For this review, take the finished solid that the model builds, in its own axes (mm). Face numbers are marked on the shaded views. A direction names the side the tool comes from. Round coordinates to 2 decimals unless told otherwise and drop trailing zeros. Loops run counter-clockwise (first coordinate to the right, second up) from the corner with the lowest first, then second, coordinate; pieces in that order, holes last.
1) Insertion check: pin 1 (18 mm diameter, centred on x = 24, z = -19, fed in from -Y). The pin has a flat end and moves straight along its axis. Give the tip position at first contact, or say it passes through.
2) Take a section at A-A (x = 32). State the section outline as (y, z) points.
3) Wall thickness on L1, parallel to Z at x = 24, y = 8; L2, parallel to X at y = 12, z = -17.5; L3, parallel to X at y = 9.25, z = -11: over which ranges is each line inside the solid? List them lowest first.
4) Take a section at B-B (z = -11). State the section outline as (x, y) points, then the cut area to 3 significant figures.
5) Tool access review of the marked faces 1 and 2: name each direction out of +Z, -Z, +X, -X, +Y, -Y from which nothing blocks a thin tool from reaching the whole face with its end or side.
6) Mouldability with a two-part tool opening along X and no side actions: class the marked faces 3, 4 and 5 as pulls with the +X half, pulls with the -X half, needs draft (parallel to the pull), parting line crosses it, or undercut.
7) Take a section at D-D (z = -21). State the section outline as (x, y) points, then the cut area to 3 significant figures.
8) Take a section at C-C (y = 4.75). State the section outline as (x, z) points.
Autodesk Inventor part; units mm, degrees
ref_plane "YZ Plane" through (0, 0, 0) normal (1, 0, 0) x (0, 1, 0)
ref_plane "XZ Plane" through (0, 0, 0) normal (0, 1, 0) x (-1, 0, 0)
ref_plane "XY Plane" through (0, 0, 0) normal (0, 0, 1) x (1, 0, 0)
sketch "Sketch1" plane through (0, 0, 0) normal (0, 1, 0) x (-1, 0, 0)
  line L0 (-84, -3) -> (-84, -35)
  line L1 (-80, -39) -> (-24, -39)
  line L2 (-52, -9) -> (-52, -23)
  line L3 (-56, -27) -> (-68, -27)
  line L4 (-72, -23) -> (-72, -3)
  line L5 (-24, 1) -> (-42, 1)
  line L6 (-76, 1) -> (-80, 1)
  arc A0 (-80, 1) -> (-84, -3) centre (-80, -3) ccw
  arc A1 (-72, -3) -> (-76, 1) centre (-76, -3) ccw
  arc A2 (-84, -35) -> (-80, -39) centre (-80, -35) ccw
  arc A3 (-72, -23) -> (-68, -27) centre (-68, -23) ccw
  arc A4 (-56, -27) -> (-52, -23) centre (-56, -23) ccw
  arc A5 (-24, -39) -> (-24, 1) centre (-24, -19) ccw
  arc A6 (-42, 1) -> (-52, -9) centre (-42, -9) ccw
  line L7 (-4, -19) -> (-4, -49)
  line L8 (-4, -49) -> (-84, -49)
  line L9 (-84, -49) -> (-84, -35)
  point P0 (-84, -39)
  point P1 (-52, -27)
  point P2 (-52, 1)
  point P3 (-72, -27)
  dimension "d2" = 20
  dimension "d4" = 12
  dimension "d6" = 40
  dimension "d9" = 40
  dimension "d24" = 4
  dimension "d25" = 10
  dimension "d26" = 28
  dimension "d27" = 12
  dimension "d32" = 30
extrude "Extrusion1" add sketch "Sketch1" along normal blind 12.7
sketch "Sketch2" plane through (0, 12.7, 0) normal (0, 1, 0) x (1, 0, 0)
  circle A0 centre (24, 19) radius 7
  arc A1 (4, 19) -> (24, -1) centre (24, 19) ccw
  circle A2 centre (32, 27) radius 2.05
  circle A3 centre (16, 27) radius 2.05
  circle A4 centre (16, 11) radius 2.05
  circle A5 centre (32, 11) radius 2.05
  point P0 (0, 0)
  point P1 (24, 39)
  dimension "d13" = 14
  dimension "d14" = 4.1
  dimension "d15" = 4.1
  dimension "d16" = 4.1
  dimension "d17" = 4.1
  dimension "d18" = 16
  dimension "d19" = 16
  dimension "d20" = 8
  dimension "d21" = 8
extrude "Extrusion2" cut sketch "Sketch2" against normal through all
fillet "Fillet1" radius 5 2 edges at (84, 6.35, -49) (4, 6.35, -49)
properties part number "platform hook"
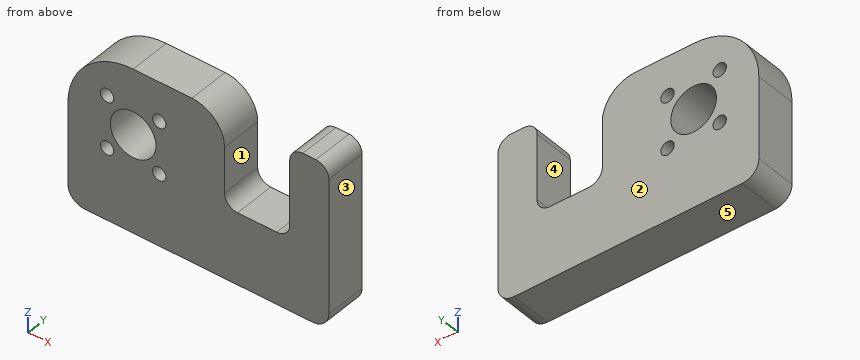
Response:
1. pin 1: stops at y = 0
2. outline: (0, -49) - (12.7, -49) - (12.7, -29.05) - (0, -29.05) - close; (0, -24.95) - (12.7, -24.95) - (12.7, -13.05) - (0, -13.05) - close; (0, -8.95) - (12.7, -8.95) - (12.7, 1) - (0, 1) - close
3. L1: z = -49 to -26, -12 to 1
3. L2: x = 4.06 to 17.16, 30.84 to 52, 72 to 84
3. L3: x = 5.67 to 13.95, 18.05 to 29.95, 34.05 to 52, 72 to 84
4. outline: (5.67, 0) - (13.95, 0) - (13.95, 12.7) - (5.67, 12.7) - close; (18.05, 0) - (29.95, 0) - (29.95, 12.7) - (18.05, 12.7) - close; (34.05, 0) - (52, 0) - (52, 12.7) - (34.05, 12.7) - close; (72, 0) - (84, 0) - (84, 12.7) - (72, 12.7) - close
4. area: 637 mm2
5. face 1: +Z, +Y, -Y
5. face 2: +Z, -Z, +X, -X, +Y
6. face 3: pulls with the +X half
6. face 4: undercut
6. face 5: needs draft
7. outline: (4, 0) - (17.29, 0) - (17.29, 12.7) - (4, 12.7) - close; (30.71, 0) - (52, 0) - (52, 12.7) - (30.71, 12.7) - close; (72, 0) - (84, 0) - (84, 12.7) - (72, 12.7) - close
7. area: 592 mm2
8. outline: (4, -44) arc R5 ccw to (9, -49) - (79, -49) arc R5 ccw to (84, -44) - (84, -3) arc R4 ccw to (80, 1) - (76, 1) arc R4 ccw to (72, -3) - (72, -23) arc R4 cw to (68, -27) - (56, -27) arc R4 cw to (52, -23) - (52, -9) arc R10 ccw to (42, 1) - (24, 1) arc R20 ccw to (4, -19) - close; hole circle Ø4.1 at (16, -27); hole circle Ø4.1 at (16, -11); hole circle Ø14 at (24, -19); hole circle Ø4.1 at (32, -27); hole circle Ø4.1 at (32, -11)
